from build123d import *

# Parameters (mm, degrees)
F0_R     = 5.5372
F0_R_2   = 4.0132
F1_DEPTH = 2.54
F3_DEPTH = 2.541
F5_DEPTH = 2.54


with BuildPart() as f1:
    # F0 (on Top) → F1 (new body)
    with BuildSketch(Plane.XY):
        Circle(F0_R)
        Circle(F0_R_2, mode=Mode.SUBTRACT)
    extrude(amount=F1_DEPTH)

    # F2 (on face) → F3 (cut, through all)
    with BuildSketch(Plane.XY.offset(2.54)):
        with BuildLine():
            ThreePointArc((-3.884592, -1.007827), (-4.0132, 0), (-3.884592, 1.007827))
            ThreePointArc((-3.884592, 1.007827), (-5.0292, 0), (-3.884592, -1.007827))
        make_face()
    extrude(amount=-F3_DEPTH, mode=Mode.SUBTRACT)

    # F4 (on face) → F5 (join, through all)
    with BuildSketch(Plane.XY.offset(2.54)):
        with BuildLine():
            ThreePointArc((-5.02277, -2.330744), (-5.5372, 0), (-5.02277, 2.330744))
            ThreePointArc((-5.02277, 2.330744), (-6.5532, 0), (-5.02277, -2.330744))
        make_face()
    extrude(amount=-F5_DEPTH)


solid = f1.part
Verification items for the finished model (mm, model axes). Give positions to 0.01 mm unless a question says otherwise; leave off trailing zeros. Order: outer loops, then holes, each group sorted by start corner. A loop starts at its lowest first (then second) coordinate and runs counter-clockwise, first axis right, second up. Notation, with made-up numbers: M -16.5,84 L -7.5,84 A21 ccw -7.5,89 Z; hole C 57.5,28 d6. An arc over 180 degrees is marked long. Answer as a JSON object with one key per item and string values. Group by question number.
1) Depth check by flat-ended pin: pin 1 Ø1 at (y, z) = (4, 1) entering from +X; pin 2 Ø1.5 at (y, z) = (1.5, 2) entering from +X. Enter the tip coordinate at first touch or a pass-through.
2) Scan lines: line 1 along Y through (x, z) = (0, 0.75); line 2 along X through (y, z) = (2.75, 1.7); line 3 along Y through (x, z) = (2.5, 0.7). Record each from-to range of solid material in increasing order. Write a range as [from, to].
3) Mould release check, pull along Y, two halves, no side actions. Record for faces 1 (the face through (5.533, -0.21, 1.252)), 2 (the face through (-3, 3, 2.54)), 3 (the face through (-5.03, 0.02, 1.29)): released by +Y, released by -Y, zero draft, split by the parting line, or undercut.
4) Cross-section at A-A (x = 0). Enter the section's corners in (y, z).
5) Cross-section at B-B (y = 0). Enter the section's corners in (x, z).
6) Cross-section at C-C (z = 0.55). Enter the section's corners in (x, y).
7) Cross-section at D-D (x = -5.5). Enter the section's corners in (y, z).
Result sheet:
{
 "1": {"pin 1": "stops at x = 4.29", "pin 2": "stops at x = 5.49"},
 "2": {"line 1": "y = [-5.54, -4.01], [4.01, 5.54]", "line 2": "x = [-4.81, -2.92], [2.92, 4.81]", "line 3": "y = [-4.94, -3.14], [3.14, 4.94]"},
 "3": {"face 1": "split by the parting line", "face 2": "zero draft", "face 3": "undercut"},
 "4": {"outline": "M -5.54,0 L -4.01,0 L -4.01,2.54 L -5.54,2.54 Z; M 4.01,0 L 5.54,0 L 5.54,2.54 L 4.01,2.54 Z"},
 "5": {"outline": "M -6.55,0 L -5.03,0 L -5.03,2.54 L -6.55,2.54 Z; M 4.01,0 L 5.54,0 L 5.54,2.54 L 4.01,2.54 Z"},
 "6": {"outline": "M -5.02,-2.33 A5.54 ccw long -5.02,2.33 A2.54 ccw Z; hole M -3.88,-1.01 A4.01 ccw long -3.88,1.01 A1.02 ccw long Z"},
 "7": {"outline": "M -2.06,0 L 2.06,0 L 2.06,2.54 L -2.06,2.54 Z"}
}
